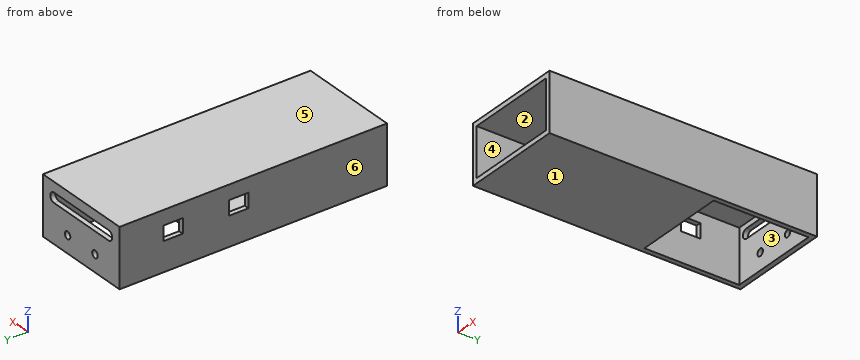
from build123d import *

# Parameters (mm, degrees)
SKETCH_1_W          = 38
SKETCH_1_H          = 106
EXTRUDE_1_DEPTH     = 2
SKETCH_2_W          = 42
SKETCH_2_H          = 110
SKETCH_2_W_2        = 38
SKETCH_2_H_2        = 39
SKETCH_2_H_3        = 65
EXTRUDE_5_DEPTH     = 24
SKETCH_9_W          = 6
SKETCH_9_H          = 8
CUT_EXTRUDE_2_DEPTH = 20
SKETCH_10_R         = 1.5
CUT_EXTRUDE_3_DEPTH = 20
SKETCH_12_W         = 38
SKETCH_12_H         = 65
EXTRUDE_7_DEPTH     = 2
SKETCH_13_W         = 38
SKETCH_13_H         = 20
CUT_EXTRUDE_4_DEPTH = 2
EXTRUDE_START       = 22
SKETCH_11_W         = 38
SKETCH_11_H         = 26.2
EXTRUDE_6_DEPTH     = 1.5


with BuildPart() as part:
    # Sketch 1 → Extrude 1 (new body)
    with BuildSketch(Plane.XY):
        with Locations((-19, 20.675324675)):
            Rectangle(SKETCH_1_W, SKETCH_1_H)
    extrude(amount=EXTRUDE_1_DEPTH)

    # Sketch 2 → Extrude 5 (add)
    with BuildSketch(Plane.XY.offset(2)):
        with Locations((-19, 20.675324675)):
            Rectangle(SKETCH_2_W, SKETCH_2_H)
        with Locations((-19, 54.175324675)):
            Rectangle(SKETCH_2_W_2, SKETCH_2_H_2, mode=Mode.SUBTRACT)
        with Locations((-19, 0.175324675)):
            Rectangle(SKETCH_2_W_2, SKETCH_2_H_3, mode=Mode.SUBTRACT)
    extrude(amount=-EXTRUDE_5_DEPTH)

    # Sketch 9 → Cut-Extrude 2 (cut)
    with BuildSketch(Plane.ZY.offset(40)):
        with Locations((-7, 26.675324675)):
            Rectangle(SKETCH_9_W, SKETCH_9_H)
        with Locations((-7, 53.675324675)):
            Rectangle(SKETCH_9_W, SKETCH_9_H)
    extrude(amount=-CUT_EXTRUDE_2_DEPTH, mode=Mode.SUBTRACT)

    # Sketch 10 → Cut-Extrude 3 (cut)
    with BuildSketch(Plane(origin=(0, 75.675324675, 0), x_dir=(1, 0, 0), z_dir=(0, 1, 0))):
        with Locations(Location((-26.5, 15, 0), (0, 0, 270))):
            Circle(SKETCH_10_R)
        with Locations(Location((-11.5, 15, 0), (0, 0, 270))):
            Circle(SKETCH_10_R)
        with BuildLine():
            Line((-34, 6.130920254), (-4, 6.130920254))
            ThreePointArc((-4, 6.130920254), (-2, 4.130920254), (-4, 2.130920254))
            Line((-4, 2.130920254), (-34, 2.130920254))
            ThreePointArc((-34, 2.130920254), (-36, 4.130920254), (-34, 6.130920254))
        make_face()
    extrude(amount=-CUT_EXTRUDE_3_DEPTH, mode=Mode.SUBTRACT)

    # Sketch 12 → Extrude 7 (add)
    with BuildSketch(Plane(origin=(0, 0, -22), x_dir=(-1, 0, 0), z_dir=(0, 0, -1))):
        with Locations((19, 0.175324675)):
            Rectangle(SKETCH_12_W, SKETCH_12_H)
    extrude(amount=-EXTRUDE_7_DEPTH)

    # Sketch 13 → Cut-Extrude 4 (cut)
    with BuildSketch(Plane.XZ.offset(34.324675325)):
        with Locations((-19, -10)):
            Rectangle(SKETCH_13_W, SKETCH_13_H)
    extrude(amount=-CUT_EXTRUDE_4_DEPTH, mode=Mode.SUBTRACT)

    # Sketch 11 → Extrude 6 (add)
    with BuildSketch(Plane(origin=(0, 0, 0), x_dir=(-1, 0, 0), z_dir=(0, 0, -1)).offset(EXTRUDE_START)):
        with Locations((19, 57.775324675)):
            Rectangle(SKETCH_11_W, SKETCH_11_H)
    extrude(amount=EXTRUDE_6_DEPTH)


with BuildPart() as extrude_6_kept_piece:
    # of the separate pieces the step leaves, the one the design keeps (extrude_6_pieces_kept)
    add(part.part.solids().sort_by_distance((-38, 34.675324675, 0))[0])


solid = extrude_6_kept_piece.part
Here's how the part is built. I have some questions about the finished solid (model axes, mm). Face numbers are marked on the shaded views. A direction names the side the tool comes from. Coordinates: 2 decimals unless noted, no trailing zeros. Write each loop counter-clockwise with the first axis right and the second up, starting at its lowest first coordinate (ties: lowest second). Pieces come first, ordered by that corner, then holes.
1) If we section it at D-D (x = -26.5): List the corners of the cut face in (y, z) for me.
Filled in:
outline: (-34.32, -22) - (34.68, -22) - (34.68, 0) - (73.68, 0) - (73.68, -2.13) - (75.68, -2.13) - (75.68, 2) - (-34.32, 2) - (-34.32, 0) - (32.68, 0) - (32.68, -20) - (-34.32, -20) - close; (73.68, -22) - (75.68, -22) - (75.68, -16.5) - (73.68, -16.5) - close; (73.68, -13.5) - (75.68, -13.5) - (75.68, -6.13) - (73.68, -6.13) - close
2) If we section it at B-B (x = -33): List the corners of the cut face in (y, z) for me.
Filled in:
outline: (-34.32, -22) - (34.68, -22) - (34.68, 0) - (73.68, 0) - (73.68, -2.13) - (75.68, -2.13) - (75.68, 2) - (-34.32, 2) - (-34.32, 0) - (32.68, 0) - (32.68, -20) - (-34.32, -20) - close; (73.68, -22) - (75.68, -22) - (75.68, -6.13) - (73.68, -6.13) - close
3) If we section it at C-C (y = 54.5): List the corners of the cut face in (x, z) for me.
Filled in:
outline: (-40, -22) - (-38, -22) - (-38, -10) - (-40, -10) - close; (-40, -4) - (-38, -4) - (-38, 0) - (0, 0) - (0, -22) - (2, -22) - (2, 2) - (-40, 2) - close
4) Thinking about a two-plate mould opening in X: for the marked faces 4, 5 and 6, which applies, +X half, -X half, draft (parallel to the pull), parting line (faces both ways), or undercut?
Filled in:
face 4: undercut
face 5: draft
face 6: -X half
5) Which directions (+Z, -Z, +X, -X, +Y, -Y) give clear straight access to the entire face, cutting with the end or side of a thin tool? Please do the marked faces 1, 2 and 3.
Filled in:
face 1: -Z, +X, -X, +Y, -Y
face 2: -Y
face 3: -Z
6) If I drill on line 1 (X direction, y = 75.2, z = -15); line 2 (Y direction, x = -16, z = -15); line 3 (Y direction, x = -11, z = -20.25), over which ranges is the centre line in solid material (lowest first)?
Filled in:
line 1: x = -40 to -28, -25 to -13, -10 to 2
line 2: y = 32.68 to 34.68, 73.68 to 75.68
line 3: y = -34.32 to 34.68, 73.68 to 75.68
7) If we section it at A-A (z = -15): List the corners of the cut face in (x, y) for me.
Filled in:
outline: (-40, -34.32) - (-38, -34.32) - (-38, 32.68) - (0, 32.68) - (0, -34.32) - (2, -34.32) - (2, 75.68) - (-10, 75.68) - (-10, 73.68) - (0, 73.68) - (0, 34.68) - (-38, 34.68) - (-38, 73.68) - (-28, 73.68) - (-28, 75.68) - (-40, 75.68) - close; (-25, 73.68) - (-13, 73.68) - (-13, 75.68) - (-25, 75.68) - close
8) I'm going to push flat-ended pins straight in: pin 1 (1.8 mm diameter, centred on x = -11.5, z = -15, fed in from +Y); pin 2 (11 mm diameter, centred on x = -25.5, z = -9.5, fed in from -Y). Where does each tip first touch, or does it pass through?
Filled in:
pin 1: stops at y = 34.68
pin 2: stops at y = 32.68
